Verification items for the finished model (mm, model axes). A direction names the side the tool comes from. Coordinates: 2 decimals unless noted, no trailing zeros. Order: outer loops, then holes, each group sorted by start corner. A loop starts at its lowest first (then second) coordinate and runs counter-clockwise, first axis right, second up. Notation, with made-up numbers: M 29.5,47 L 66.5,47 A19 cw 66.5,64 Z; hole C 66,9 d11. An arc over 180 degrees is marked long. Return JSON: item names as keys, results as strings. Group by question number.
Q1. Section check A-A, the plane z = 305. Enter the section's corners in (x, y), then the cut area to 3 significant figures.
Q2. Go/stop test with flat-tipped pins: pin 1 Ø5 at (x, y) = (53, -60) entering from +Z; pin 2 Ø5 at (x, y) = (40.5, -45) entering from -Z; pin 3 Ø6 at (x, y) = (25.5, -111.5) entering from +Z. Record where each tip stops, or that it passes through.
Q3. Thickness scan on probe 1 along Y at (x, z) = (10, 313); probe 2 along Z at (x, y) = (50.5, -86); probe 3 along Z at (x, y) = (5.5, -36). Record the ranges inside material, lowest first.
Q4. Access from +Z, -Z, +X, -X, +Y, -Y to the whole of each face (thin tool, end or side, straight path). Record for faces 5 (the face through (29.58, -87.027, 860.222)), 6 (the face through (29.58, -87.36, 875.22)).
Q5. Mould release check, pull along Y, two halves, no side actions. Record for faces 1 (the face through (30, -150.598, 369)), 2 (the face through (30, -20.598, 381)), 3 (the face through (30, -87, -126)), 4 (the face through (30, -5.598, 381)): pulls with the +Y half, pulls with the -Y half, needs draft (parallel to the pull), parting line crosses it, or undercut.
Q6. Section check C-C, the plane y = -49. Enter the section's corners in (x, z), then the cut area to 3 significant figures.
Q7. Section check B-B, the plane x = 39. Enter the section's corners in (y, z).
from build123d import *

# Parameters (mm, degrees)
SKETCH_1_R               = 18.541316536
EXTRUDE_1_DEPTH          = 10
SKETCH_2_R               = 65
EXTRUDE_2_DEPTH          = 60
CUT_EXTRUDE_1_DEPTH      = 554.983106248
CUT_EXTRUDE_1_DEPTH_BACK = 554.983106248
CUT_EXTRUDE_2_DEPTH      = 554.983106248
CUT_EXTRUDE_2_DEPTH_BACK = 554.983106248
SKETCH_4_W               = 491.25
SKETCH_4_H               = 130
EXTRUDE_START            = -60
EXTRUDE_3_DEPTH          = 60
CUT_EXTRUDE_3_DEPTH      = 229


with BuildPart() as part:
    # 草图1 → 凸台-拉伸1 (new body)
    with BuildSketch(Plane(origin=(0, 0, 0), x_dir=(0, 0, -1), z_dir=(1, 0, 0))):
        Circle(SKETCH_1_R)
    extrude(amount=EXTRUDE_1_DEPTH)

    # 草图2 → 凸台-拉伸2 (add)
    with BuildSketch(Plane.ZY):
        with BuildLine():
            Line((-46.012206562, -5.59753124), (445.237793438, -5.59753124))
            ThreePointArc((445.237793438, -5.59753124), (525.237793438, -85.59753124), (445.237793438, -165.59753124))
            Line((445.237793438, -165.59753124), (-46.012206562, -165.59753124))
            ThreePointArc((-46.012206562, -165.59753124), (-126.012206562, -85.59753124), (-46.012206562, -5.59753124))
        make_face()
        with Locations((-46.012206562, -85.59753124)):
            Circle(SKETCH_2_R, mode=Mode.SUBTRACT)
        with Locations((445.237793438, -85.59753124)):
            Circle(SKETCH_2_R, mode=Mode.SUBTRACT)
    extrude(amount=-EXTRUDE_2_DEPTH)

    # 草图3 → 切除-拉伸1 (cut, two sides: drawn at the far end of the back side and taken through both)
    with BuildSketch(Plane.ZY.offset(-CUT_EXTRUDE_1_DEPTH_BACK)):
        Polygon((-32.271946136, -5.59753124), (45.25223132, -5.59753124), (36.799677621, 39.571185564), (-16.420104924, 39.571185564), align=None)
    extrude(amount=CUT_EXTRUDE_1_DEPTH + CUT_EXTRUDE_1_DEPTH_BACK, mode=Mode.SUBTRACT)

    # 草图4 → 切除-拉伸2 (cut, two sides: drawn at the far end of the back side and taken through both)
    with BuildSketch(Plane.ZY.offset(-CUT_EXTRUDE_2_DEPTH_BACK)):
        with Locations((199.612793438, -85.59753124)):
            Rectangle(SKETCH_4_W, SKETCH_4_H)
    extrude(amount=CUT_EXTRUDE_2_DEPTH + CUT_EXTRUDE_2_DEPTH_BACK, mode=Mode.SUBTRACT)

    # 草图6 → 凸台-拉伸3 (add)
    with BuildSketch(Plane(origin=(60, 0, 0), x_dir=(0, 0, -1), z_dir=(1, 0, 0)).offset(EXTRUDE_START)):
        with BuildLine():
            Line((-795.237793438, -5.59753124), (46.012206562, -5.59753124))
            ThreePointArc((46.012206562, -5.59753124), (126.012206562, -85.59753124), (46.012206562, -165.59753124))
            Line((46.012206562, -165.59753124), (-795.237793438, -165.59753124))
            ThreePointArc((-795.237793438, -165.59753124), (-875.237793438, -85.59753124), (-795.237793438, -5.59753124))
        make_face()
        with BuildLine():
            Line((-795.237793438, -20.59753124), (46.012206562, -20.59753124))
            ThreePointArc((46.012206562, -20.59753124), (111.012206562, -85.59753124), (46.012206562, -150.59753124))
            Line((46.012206562, -150.59753124), (-795.237793438, -150.59753124))
            ThreePointArc((-795.237793438, -150.59753124), (-860.237793438, -85.59753124), (-795.237793438, -20.59753124))
        make_face(mode=Mode.SUBTRACT)
    extrude(amount=EXTRUDE_3_DEPTH)

    # 草图7 → 切除-拉伸3 (cut)
    with BuildSketch(Plane(origin=(60, 0, 0), x_dir=(0, 0, -1), z_dir=(1, 0, 0))):
        Polygon((-547.566166751, -20.59753124), (-408.942471001, -20.59753124), (-408.942471001, -150.59753124), (-543.921935574, -150.59753124), align=None)
    extrude(amount=-CUT_EXTRUDE_3_DEPTH, mode=Mode.SUBTRACT)


solid = part.part
Numbers:
{
 "1": {"outline": "M 0,-165.6 L 60,-165.6 L 60,-150.6 L 0,-150.6 Z; M 0,-20.6 L 60,-20.6 L 60,-5.6 L 0,-5.6 Z", "area": "1,800 mm2"},
 "2": {"pin 1": "stops at z = 871.83", "pin 2": "stops at z = -116.36", "pin 3": "stops at z = 871.89"},
 "3": {"probe 1": "y = -165.6 to -150.6, -20.6 to -5.6", "probe 2": "z = -126.01 to -111.01, 860.24 to 875.24", "probe 3": "z = -108.78 to -88.03, 837.25 to 858.01"},
 "4": {"face 5": "+X, -X", "face 6": "+Z, +X, -X"},
 "5": {"face 1": "undercut", "face 2": "undercut", "face 3": "parting line crosses it", "face 4": "pulls with the +Y half"},
 "6": {"outline": "M 0,-117.15 L 60,-117.15 L 60,-99.73 L 0,-99.73 Z; M 0,848.96 L 60,848.96 L 60,866.38 L 0,866.38 Z", "area": "2,090 mm2"},
 "7": {"outline": "M -165.6,-46.01 A80 ccw -5.6,-46.01 L -5.6,795.24 A80 ccw -165.6,795.24 Z; hole M -150.6,-46.01 A65 ccw -20.6,-46.01 L -20.6,795.24 A65 ccw -150.6,795.24 Z"}
}
